Verification items for the finished model (mm, model axes). Coordinates: 2 decimals unless noted, no trailing zeros. Write each loop counter-clockwise with the first axis right and the second up, starting at its lowest first coordinate (ties: lowest second). Pieces come first, ordered by that corner, then holes. Notation, with made-up numbers: (54.25, -17) -> (60.25, -17) arc R23 cw to (60.25, 9) -> close; hole circle Ø2 at (55, 12). An arc over 180 degrees is marked (long way). Write item = value, one per line. Start each with the question number.
(1) Section check B-B (z = 0). Record the cut outline in (x, y), plus the area to 3 significant figures.
(2) Material ranges on probe 1 along X at (y, z) = (2.8, 0); probe 2 along X at (y, z) = (0.6, -19.5); probe 3 along X at (y, z) = (4.6, 22), recorded low to high. Write a range as [from, to].
(3) Gauge pin test, flat ends, axial feed: pin 1 Ø2 at (x, z) = (25, 0) entering from +Y; pin 2 Ø1.5 at (x, y) = (-30.5, 2) entering from -Z. Record the tip position at first contact, or that the pin passes through.
(4) Mould release check, pull along X, two halves, no side actions. Record for faces 1 (the face through (-23, 0, -1)), 2 (the face through (-33.693, 3.042, -26.379)), 3 (the face through (-53.204, 2.958, -11.815)): released by +X, released by -X, zero draft, split by the parting line, or undercut.
(5) Section check C-C (y = 4). Record the cut outline in (x, z).
(6) Section check D-D (z = 25). Record the cut outline in (x, y).
(7) Section check A-A (x = 0). Record the cut outline in (y, z), plus the area to 3 significant figures.
```python
from build123d import *

# Parameters (mm, degrees)
SKETCH_1_R          = 54.5
EXTRUDE_1_DEPTH     = 6
SKETCH_2_R          = 2.5
CUT_EXTRUDE_1_DEPTH = 6
SKETCH_3_R          = 18.5
SKETCH_3_R_2        = 1.65
CUT_EXTRUDE_2_DEPTH = 6


with BuildPart() as part:
    # Эскиз1 → Бобышка-Вытянуть1 (new body)
    with BuildSketch(Plane(origin=(0, 0, 0), x_dir=(1, 0, 0), z_dir=(0, 1, 0))):
        with Locations(Location((0, 0, 0), (0, 0, 270))):
            Circle(SKETCH_1_R)
    extrude(amount=EXTRUDE_1_DEPTH)

    # Эскиз2 → Вырез-Вытянуть1 (cut)
    with BuildSketch(Plane(origin=(0, 6, 0), x_dir=(1, 0, 0), z_dir=(0, 1, 0))):
        with Locations(Location((0, 42.5, 0), (0, 0, 270))):
            Circle(SKETCH_2_R)
        with BuildLine():
            ThreePointArc((-42.002232084, 24.25), (0, -48.5), (42.002232084, 24.25))
            ThreePointArc((42.002232084, 24.25), (33.806079661, 26.446152423), (31.609927238, 18.25))
            ThreePointArc((31.609927238, 18.25), (0, -36.5), (-31.609927238, 18.25))
            ThreePointArc((-31.609927238, 18.25), (-33.806079661, 26.446152423), (-42.002232084, 24.25))
        make_face()
    extrude(amount=-CUT_EXTRUDE_1_DEPTH, mode=Mode.SUBTRACT)

    # Эскиз3 → Вырез-Вытянуть2 (cut)
    with BuildSketch(Plane(origin=(0, 6, 0), x_dir=(1, 0, 0), z_dir=(0, 1, 0))):
        with Locations(Location((0, 0, 0), (0, 0, 270))):
            Circle(SKETCH_3_R)
        with Locations(Location((0, 25, 0), (0, 0, 270))):
            Circle(SKETCH_3_R_2)
        with Locations(Location((-25, 0, 0), (0, 0, 270))):
            Circle(SKETCH_3_R_2)
        with Locations(Location((0, -25, 0), (0, 0, 270))):
            Circle(SKETCH_3_R_2)
        with Locations(Location((25, 0, 0), (0, 0, 270))):
            Circle(SKETCH_3_R_2)
    extrude(amount=-CUT_EXTRUDE_2_DEPTH, mode=Mode.SUBTRACT)


solid = part.part
```
Response:
q1.outline = (-54.5, 0) -> (-48.5, 0) -> (-48.5, 6) -> (-54.5, 6) -> close; (-36.5, 0) -> (-26.65, 0) -> (-26.65, 6) -> (-36.5, 6) -> close; (-23.35, 0) -> (-18.5, 0) -> (-18.5, 6) -> (-23.35, 6) -> close; (18.5, 0) -> (23.35, 0) -> (23.35, 6) -> (18.5, 6) -> close; (26.65, 0) -> (36.5, 0) -> (36.5, 6) -> (26.65, 6) -> close; (48.5, 0) -> (54.5, 0) -> (54.5, 6) -> (48.5, 6) -> close
q1.area = 248 mm2
q2.probe_1 = [-54.5, -48.5], [-36.5, -26.65], [-23.35, -18.5], [18.5, 23.35], [26.65, 36.5], [48.5, 54.5]
q2.probe_2 = [-50.89, -44.41], [-31.07, 31.07], [44.41, 50.89]
q2.probe_3 = [-49.86, -43.22], [-29.12, 29.12], [43.22, 49.86]
q3.pin_1 = through
q3.pin_2 = -45.66
q4.face_1 = zero draft
q4.face_2 = undercut
q4.face_3 = split by the parting line
q5.outline = circle Ø109 at (0, 0); hole (-42, -24.25) arc R6 ccw to (-31.61, -18.25) arc R36.5 cw (long way) to (31.61, -18.25) arc R6 ccw to (42, -24.25) arc R48.5 ccw (long way) to start; hole circle Ø3.3 at (-25, 0); hole circle Ø37 at (0, 0); hole circle Ø5 at (0, -42.5); hole circle Ø3.3 at (0, -25); hole circle Ø3.3 at (0, 25); hole circle Ø3.3 at (25, 0)
q6.outline = (-48.43, 0) -> (-41.56, 0) -> (-41.56, 6) -> (-48.43, 6) -> close; (-26.59, 0) -> (-1.65, 0) -> (-1.65, 6) -> (-26.59, 6) -> close; (1.65, 0) -> (26.59, 0) -> (26.59, 6) -> (1.65, 6) -> close; (41.56, 0) -> (48.43, 0) -> (48.43, 6) -> (41.56, 6) -> close
q7.outline = (0, -54.5) -> (6, -54.5) -> (6, -45) -> (0, -45) -> close; (0, -40) -> (6, -40) -> (6, -26.65) -> (0, -26.65) -> close; (0, -23.35) -> (6, -23.35) -> (6, -18.5) -> (0, -18.5) -> close; (0, 18.5) -> (6, 18.5) -> (6, 23.35) -> (0, 23.35) -> close; (0, 26.65) -> (6, 26.65) -> (6, 36.5) -> (0, 36.5) -> close; (0, 48.5) -> (6, 48.5) -> (6, 54.5) -> (0, 54.5) -> close
q7.area = 290 mm2
